```python
from build123d import *

# Parameters (mm, degrees)
EXTRUDE_1_DEPTH             = 6
CUT_EXTRUDE_1_DEPTH         = 7
HOLE_WIZARD_9_0_9_1_D       = 9
HOLE_WIZARD_9_0_9_1_DEPTH   = 6
HOLE_WIZARD_3_2_3_2_1_D     = 3.2
HOLE_WIZARD_3_2_3_2_1_DEPTH = 6
FILLET_1_R                  = 5
CHAMFER_1_SIZE              = 0.5


with BuildPart() as part:
    # 草图1 → 凸台-拉伸1 (new body)
    with BuildSketch(Plane.XY.offset(6)):
        with BuildLine():
            Line((-54.404710274, 17.5), (-58.249656651, 15))
            ThreePointArc((-58.249656651, 15), (0, -60.15), (58.249656651, 15))
            Line((58.249656651, 15), (54.404710274, 17.5))
            ThreePointArc((54.404710274, 17.5), (0, 57.15), (-54.404710274, 17.5))
        make_face()
    extrude(amount=-EXTRUDE_1_DEPTH)

    # 草图2 → 切除-拉伸1 (cut, through all)
    with BuildSketch(Plane(origin=(0, 0, 0), x_dir=(-1, 0, 0), z_dir=(0, 0, -1))):
        with BuildLine():
            Line((58.249656651, -15), (54.404710274, -17.5))
            ThreePointArc((54.404710274, -17.5), (0, -57.15), (-54.404710274, -17.5))
            Line((-54.404710274, -17.5), (-58.249656651, -15))
            ThreePointArc((-58.249656651, -15), (0, -60.15), (58.249656651, -15))
        make_face()
    extrude(amount=-CUT_EXTRUDE_1_DEPTH, mode=Mode.SUBTRACT)

    # Ø9.0 (9) 直径孔1
    with Locations(Plane(origin=(0, 0, 0), x_dir=(-1, 0, 0), z_dir=(0, 0, -1))):
        with Locations((-15, 25.980762114), (15, 25.980762114), (30, 0), (15, -25.980762114), (-15, -25.980762114), (-30, 0)):
            Hole(HOLE_WIZARD_9_0_9_1_D / 2, depth=HOLE_WIZARD_9_0_9_1_DEPTH)

    # Ø3.2 (3.2) 直径孔1
    with Locations(Plane(origin=(0, 0, 0), x_dir=(-1, 0, 0), z_dir=(0, 0, -1))):
        with Locations((0, 53.975), (46.743721169, -26.9875), (-46.743721169, 26.9875), (-46.743721169, -26.9875), (0, -53.975), (46.743721169, 26.9875)):
            Hole(HOLE_WIZARD_3_2_3_2_1_D / 2, depth=HOLE_WIZARD_3_2_3_2_1_DEPTH)

    # 圆角1
    fillet_1_edges = [part.edges().sort_by_distance(p)[0] for p in [
        (-58.249656651, -15, 3),
        (58.249656651, -15, 3),
        (54.404710274, -17.5, 3),
        (-54.404710274, -17.5, 3),
        (54.404710274, 17.5, 3),
        (58.249656651, 15, 3),
        (-58.249656651, 15, 3),
        (-54.404710274, 17.5, 3),
    ]]
    fillet(fillet_1_edges, radius=FILLET_1_R)

    # 倒角1
    chamfer_1_edges = [part.edges().sort_by_distance(p)[0] for p in [
        (60.15, 0, 0),
        (56.218559502, 16.320627747, 0),
        (56.218559502, -16.320627747, 0),
        (-60.15, 0, 0),
        (-56.218559502, 16.320627747, 0),
        (0, 57.15, 0),
        (-57.961950962, 14.742761538, 0),
        (57.961950962, -14.742761538, 0),
        (-57.961950962, -14.742761538, 0),
        (57.961950962, 14.742761538, 0),
        (-54.657828511, -17.651398409, 0),
        (54.657828511, -17.651398409, 0),
        (54.657828511, 17.651398409, 0),
        (-54.657828511, 17.651398409, 0),
        (0, -57.15, 0),
        (-56.218559502, -16.320627747, 0),
    ]]
    chamfer(chamfer_1_edges, length=CHAMFER_1_SIZE)


solid = part.part
```
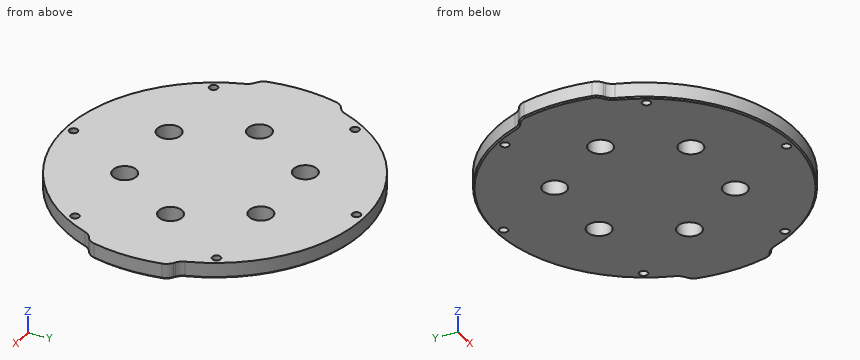
Geometry check sheet. Reference: the model listing, model coordinates, mm. Round coordinates to 2 decimals unless told otherwise and drop trailing zeros. Loops run counter-clockwise (first coordinate to the right, second up) from the corner with the lowest first, then second, coordinate; pieces in that order, holes last. Notation, with made-up numbers: M -4.5,6.5 L 1.5,6.5 A26 cw 1.5,26.5 Z; hole C -37,49.5 d2. An arc over 180 degrees is marked long. Return JSON: item names as keys, results as strings. Group by question number.
(1) Scan lines: line 1 along X through (y, z) = (-0.5, 3); line 2 along Y through (x, z) = (0, 4.7) (3 decimals); line 3 along Y through (x, z) = (15, 2.2). Record each from-to range of solid material in increasing order. Write a range as [from, to].
(2) Section check C-C, the plane z = 2.5. Give the number of separate pieces and of enclosed holes in the cut face, and give its area (3 significant figures).
(3) Section check A-A, the plane y = 0. Enter the section's corners in (x, z), and give its area (3 significant figures).
(4) Section check B-B, the plane x = 0. Enter the section's corners in (y, z) (3 decimals).
(5) Go/stop test with flat-tipped pins: pin 1 (1 mm diameter, centred on x = -5.5, z = 5, fed in from -Y); pin 2 (1 mm diameter, centred on x = -32, z = 1.5, fed in from +Y); pin 3 (14.5 mm diameter, centred on x = -15, y = -25.98, fed in from -Z); pin 4 (1 mm diameter, centred on y = -22.5, z = 1.5, fed in from +X). Record where each tip stops, or that it passes through.
Data:
{
 "1": {"line 1": "[-60.15, -34.47], [-25.53, 25.53], [34.47, 60.15]", "line 2": "[-57.15, -55.575], [-52.375, 52.375], [55.575, 57.15]", "line 3": "[-55.15, -30.48], [-21.48, 21.48], [30.48, 55.15]"},
 "2": {"separate pieces": "1", "enclosed holes": "12", "area": "10,000 mm²"},
 "3": {"outline": "M -60.15,0.5 L -59.65,0 L -34.5,0 L -34.5,6 L -60.15,6 Z; M -25.5,0 L 25.5,0 L 25.5,6 L -25.5,6 Z; M 34.5,0 L 59.65,0 L 60.15,0.5 L 60.15,6 L 34.5,6 Z", "area": "614 mm²"},
 "4": {"outline": "M -57.15,0.5 L -56.65,0 L -55.575,0 L -55.575,6 L -57.15,6 Z; M -52.375,0 L 52.375,0 L 52.375,6 L -52.375,6 Z; M 55.575,0 L 56.65,0 L 57.15,0.5 L 57.15,6 L 55.575,6 Z"},
 "5": {"pin 1": "y = -56.93", "pin 2": "y = 47.69", "pin 3": "z = 0", "pin 4": "x = 52.75"}
}
